Verification items for the finished model (mm, model axes). A direction names the side the tool comes from. Coordinates: 2 decimals unless noted, no trailing zeros. Write each loop counter-clockwise with the first axis right and the second up, starting at its lowest first coordinate (ties: lowest second). Pieces come first, ordered by that corner, then holes. Notation, with made-up numbers: M -12,-15.5 L 29,-15.5 A34 ccw 29,17.5 Z; hole C 80,73.25 d1. An arc over 180 degrees is marked long. Answer in a Markdown table with one row per item.
from build123d import *

# Parameters (mm, degrees)
F1_DEPTH = 25
F3_D     = 6.8
F3_DEPTH = 14
F3_TIP   = 2.0429261047
F4_DEPTH = 10
F5_W     = 50
F5_H     = 15
F6_DEPTH = 0.75


with BuildPart() as f1:
    # F0 (on Front) → F1 (new body)
    with BuildSketch(Plane.XZ):
        Polygon((30, 60), (0, 60), (-30, 60), (-30, 10), (-45, 10), (-45, 0), (-20, 0), (-20, 50), (0, 50), (20, 50), (20, 0), (45, 0), (45, 10), (30, 10), align=None)
    extrude(amount=F1_DEPTH)

    # F3
    with Locations(Plane.XY.offset(60)):
        with Locations((0, -12.5)):
            Hole(F3_D / 2, depth=F3_DEPTH)
            with Locations((0, 0, -(F3_DEPTH + F3_TIP / 2))):  # 118° drill point
                Cone(0, F3_D / 2, F3_TIP, mode=Mode.SUBTRACT)

    # F4 (add): a face of the model
    f4_faces = [f1.faces().sort_by_distance(p)[0] for p in [
        (29.35, -12.5, 60),
    ]]
    extrude(f4_faces, amount=F4_DEPTH)

    # F5 (on face) → F6 (cut)
    with BuildSketch(Plane.XZ.offset(25)):
        with Locations((0, 60)):
            Rectangle(F5_W, F5_H)
    extrude(amount=-F6_DEPTH, mode=Mode.SUBTRACT)


solid = f1.part
1) Thickness scan on L1, parallel to X at y = -15.5, z = 20; L2, parallel to Y at x = 0, z = 56.25; L3, parallel to Z at x = -37.5, y = -20.5. Record the ranges inside material, lowest first. Write a range as [from, to].
Response values:
| item | result |
|---|---|
| L1 | x = [-30, -20], [20, 30] |
| L2 | y = [-24.25, -15.9], [-9.1, 0] |
| L3 | z = [0, 10] |
2) Sectioned sample at C-C (y = -12.5). Record the cut outline in (x, z), then the cut area to 3 significant figures.
Response values:
| item | result |
|---|---|
| outline | M -45,0 L -20,0 L -20,50 L -3.4,50 L -3.4,70 L -30,70 L -30,10 L -45,10 Z; M 3.4,50 L 20,50 L 20,0 L 45,0 L 45,10 L 30,10 L 30,70 L 3.4,70 Z |
| area | 2,360 mm² |
3) Sectioned sample at A-A (x = 0). Record the cut outline in (y, z).
Response values:
| item | result |
|---|---|
| outline | M -25,50 L -15.9,50 L -15.9,70 L -25,70 L -25,67.5 L -24.25,67.5 L -24.25,52.5 L -25,52.5 Z; M -9.1,50 L 0,50 L 0,70 L -9.1,70 Z |
4) Release check for a two-part mould opening along Y. For faces 1 (the face through (-20, -12, 25)), 2 (the face through (0, -24.25, 60)), 3 (the face through (0.74, -15.82, 59.86)), 4 (the face through (1, 0, 58)) record: +Y half, -Y half, draft (parallel to the pull), parting line (faces both ways), or undercut.
Response values:
| item | result |
|---|---|
| face 1 | draft |
| face 2 | -Y half |
| face 3 | undercut |
| face 4 | +Y half |
5) Tool access check on faces 5 (the face through (20, -12, 25)), 6 (the face through (-30, -12, 40)), 7 (the face through (30, -12, 40)). Record the directions out of +Z, -Z, +X, -X, +Y, -Y that give a thin tool (end or side, any length) a straight path to the whole face; none if there is none.
Response values:
| item | result |
|---|---|
| face 5 | -Z, +Y, -Y |
| face 6 | +Z, -X, +Y, -Y |
| face 7 | +Z, +X, +Y, -Y |
6) Depth check by flat-ended pin: pin 1 (3 mm diameter, centred on x = -7.5, y = -5.5, fed in from -Z); pin 2 (12 mm diameter, centred on x = 40.5, y = -17, fed in from +Z); pin 3 (3 mm diameter, centred on y = -14, z = 49, fed in from -X); pin 4 (4 mm diameter, centred on x = 27, z = 26.5, fed in from +Y). Enter the tip coordinate at first touch or a pass-through.
Response values:
| item | result |
|---|---|
| pin 1 | stops at z = 50 |
| pin 2 | stops at z = 10 |
| pin 3 | stops at x = -30 |
| pin 4 | stops at y = 0 |
7) Sectioned sample at D-D (y = -17.25). Record the cut outline in (x, z), then the cut area to 3 significant figures.
Response values:
| item | result |
|---|---|
| outline | M -45,0 L -20,0 L -20,50 L 20,50 L 20,0 L 45,0 L 45,10 L 30,10 L 30,70 L -30,70 L -30,10 L -45,10 Z |
| area | 2,500 mm² |
8) Sectioned sample at B-B (z = 16). Record the cut outline in (x, y), then the cut area to 3 significant figures.
Response values:
| item | result |
|---|---|
| outline | M -30,-25 L -20,-25 L -20,0 L -30,0 Z; M 20,-25 L 30,-25 L 30,0 L 20,0 Z |
| area | 500 mm² |
